Source: CAD feature listing. Evaluate the final solid. Frame: model axes, mm. Face numbers are marked on the shaded views. A direction names the side the tool comes from. Coordinates: 2 decimals unless noted, no trailing zeros. Order: outer loops, then holes, each group sorted by start corner. A loop starts at its lowest first (then second) coordinate and runs counter-clockwise, first axis right, second up.
```python
from build123d import *

# Parameters (mm, degrees)
F0_W      = 99.06
F0_H      = 101.6
F1_DEPTH  = 45.72
F2_W      = 45.8418870593
F2_H      = 107.1278404426
F3_DEPTH  = 35.56
F4_W      = 96.4650140689
F4_H      = 66.04
F5_DEPTH  = 45.721
F6_R      = 22.85999
F7_R      = 7.9375
F8_DEPTH  = 101.601
F9_R      = 5.08
F10_R     = 10.16
F11_R     = 5.1562
F12_DEPTH = 60.961
F13_R     = 5.1562
F14_DEPTH = 10.161


# Not quite as in the source:
# - a fillet or chamfer is up to 0.001 mm smaller than in the source, because OpenCascade refuses the exact size


with BuildPart() as f1:
    # F0 (on Front) → F1 (new body)
    with BuildSketch(Plane.XZ):
        with Locations((5.5195279419, -10.1849297343)):
            Rectangle(F0_W, F0_H)
    extrude(amount=F1_DEPTH)

    # F2 (on face) → F3 (cut)
    with BuildSketch(Plane.XZ.offset(45.72)):
        with Locations((39.8704714716, -9.8085980862)):
            Rectangle(F2_W, F2_H)
    extrude(amount=-F3_DEPTH, mode=Mode.SUBTRACT)

    # F4 (on face) → F5 (cut, through all)
    with BuildSketch(Plane.XZ.offset(45.72)):
        with Locations((-41.4429790925, -10.1849297343)):
            Rectangle(F4_W, F4_H)
    extrude(amount=-F5_DEPTH, mode=Mode.SUBTRACT)

    # F6 (radius 22.86 in the source; OpenCascade refuses exactly that, so slightly less here)
    f6_edges = [f1.edges().sort_by_distance(p)[0] for p in [
        (-44.010472, 0, 31.72507),
        (-44.010472, -45.72, 31.72507),
        (-44.010472, 0, -52.09493),
        (-44.010472, -45.72, -52.09493),
    ]]
    fillet(f6_edges, radius=F6_R)

    # F7 (on face) → F8 (cut, through all)
    with BuildSketch(Plane.XY.offset(40.6150702657)):
        with Locations((-21.1504720581, -22.86)):
            Circle(F7_R)
    extrude(amount=-F8_DEPTH, mode=Mode.SUBTRACT)

    # F9
    f9_edges = [f1.edges().sort_by_distance(p)[0] for p in [
        (6.789528, -22.86, 22.83507),
        (6.789528, -22.86, -43.20493),
    ]]
    fillet(f9_edges, radius=F9_R)

    # F10
    f10_edges = [f1.edges().sort_by_distance(p)[0] for p in [
        (55.049528, -5.08, 40.61507),
        (55.049528, -5.08, -60.98493),
    ]]
    fillet(f10_edges, radius=F10_R)

    # F11 (on face) → F12 (cut, through all)
    with BuildSketch(Plane.YZ.offset(16.9495279419)):
        with Locations((-27.94, -10.1849297343)):
            Circle(F11_R)
    extrude(amount=-F12_DEPTH, mode=Mode.SUBTRACT)

    # F13 (on face) → F14 (cut, through all)
    with BuildSketch(Plane.XZ.offset(10.16)):
        with Locations((30.9195279419, 25.3750702657)):
            Circle(F13_R)
        with Locations((30.9195279419, -45.7449297343)):
            Circle(F13_R)
    extrude(amount=-F14_DEPTH, mode=Mode.SUBTRACT)


solid = f1.part
```
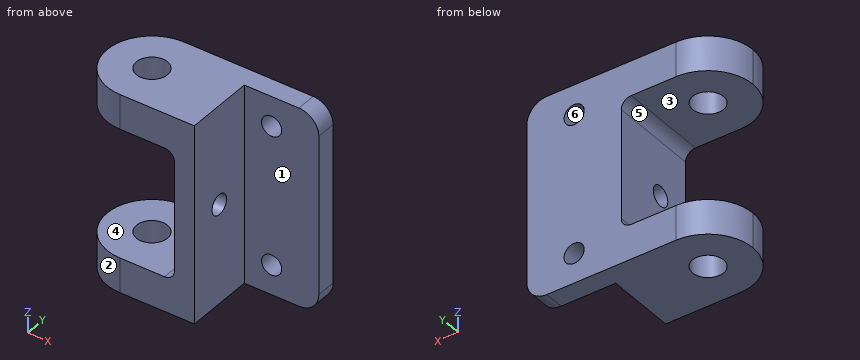
1. Draft query along X for the marked faces 4, 5 and 6. Return one class per face: released by +X, released by -X, zero draft, split by the parting line, or undercut.
Findings:
face 4: zero draft
face 5: released by -X
face 6: undercut
2. Pin query (flat end, axial travel): P1, Ø14.5, axis at x = -21.15, y = -22.86, coming from the +Z side; P2, Ø12, axis at y = -11.5, z = 16, coming from the -X side; P3, Ø6, axis at y = -33.5, z = -38, coming from the +X side; P4, Ø1, axis at x = 17.5, z = -47.5, coming from the -Y side. Return the tip coordinate at first contact, or that it passes through.
Findings:
P1: passes through
P2: stops at x = 4.5
P3: stops at x = 16.95
P4: stops at y = -10.16
3. Section query C-C on y = -20. Return loops of the section in (x, z).
Findings:
outline: (-43.83, -60.98) - (-28.55, -60.98) - (-28.55, -43.2) - (-43.83, -43.2) - close; (-43.83, 22.84) - (-28.55, 22.84) - (-28.55, 40.62) - (-43.83, 40.62) - close; (-13.75, -60.98) - (16.95, -60.98) - (16.95, 40.62) - (-13.75, 40.62) - (-13.75, 22.84) - (1.71, 22.84) arc R5.08 cw to (6.79, 17.76) - (6.79, -38.12) arc R5.08 cw to (1.71, -43.2) - (-13.75, -43.2) - close
4. Section query A-A on x = -3.5. Return loops of the section in (y, z), plus the area to 3 significant figures.
Findings:
outline: (-45.72, -60.98) - (0, -60.98) - (0, -43.2) - (-45.72, -43.2) - close; (-45.72, 22.84) - (0, 22.84) - (0, 40.62) - (-45.72, 40.62) - close
area: 1,630 mm2
5. Ray query, line 1 (Z direction, x = 13, y = -28.5); line 2 (Z direction, x = -4, y = -3); line 3 (Y direction, x = -21, z = 23.5). Return the intervals inside material, ascending.
Findings:
line 1: z = -60.98 to -15.31, -5.06 to 40.62
line 2: z = -60.98 to -43.2, 22.84 to 40.62
line 3: y = -45.72 to -30.8, -14.92 to 0
6. Section query B-B on z = 27.5. Count the separate pieces of the cut face and the enclosed holes in it, plus the area to 3 significant figures.
Findings:
separate pieces: 2
enclosed holes: 1
area: 2,660 mm2
7. Access query for the marked faces 1, 2 and 3. Directions: +Z, -Z, +X, -X, +Y, -Y. A direction counts if a zero-diameter tool reaches every point of the face in a straight line with its end or side. Return the directions, or none.
Findings:
face 1: +Z, -Z, +X, -Y
face 2: +Z, -Z, -X, -Y
face 3: -X, +Y, -Y
8. Section query D-D on x = 33. Return loops of the section in (y, z), plus the area to 3 significant figures.
Findings:
outline: (-10.16, -60.98) - (0, -60.98) - (0, -50.46) - (-10.16, -50.46) - close; (-10.16, -41.03) - (0, -41.03) - (0, 20.66) - (-10.16, 20.66) - close; (-10.16, 30.09) - (0, 30.09) - (0, 40.62) - (-10.16, 40.62) - close
area: 841 mm2
